from build123d import *

# Parameters (mm, degrees)
F2_R     = 9.525
F3_DEPTH = 1514.476


with BuildPart() as f1:
    # F0 (on Front) → F1 (revolve)
    with BuildSketch(Plane.XZ):
        Polygon((109.601, 15.875), (109.601, 0), (142.875, 0), (142.875, 25.4), (117.475, 25.4), (117.475, 22.225), (101.6, 22.225), (101.6, 15.875), align=None)
        Polygon((109.601, -1463.675), (109.601, 0), (109.601, 15.875), (101.6, 15.875), (101.6, -1479.55), (109.601, -1479.55), align=None)
        Polygon((144.526, -1463.675), (109.601, -1463.675), (109.601, -1479.55), (101.6, -1479.55), (101.6, -1485.9), (119.126, -1485.9), (119.126, -1489.075), (144.526, -1489.075), align=None)
    revolve(axis=Axis((0, 0, 9.743357), (0, 0, -1)))

    # F2 (on face) → F3 (cut, through all)
    with BuildSketch(Plane.XY.offset(25.4)):
        with Locations((130.175, 0)):
            Circle(F2_R)
        with Locations((112.734857, 65.0875)):
            Circle(F2_R)
        with Locations((65.0875, 112.734857)):
            Circle(F2_R)
        with Locations((0, 130.175)):
            Circle(F2_R)
        with Locations((-65.0875, 112.734857)):
            Circle(F2_R)
        with Locations((-112.734857, 65.0875)):
            Circle(F2_R)
        with Locations((-130.175, 0)):
            Circle(F2_R)
        with Locations((-112.734857, -65.0875)):
            Circle(F2_R)
        with Locations((-65.0875, -112.734857)):
            Circle(F2_R)
        with Locations((0, -130.175)):
            Circle(F2_R)
        with Locations((65.0875, -112.734857)):
            Circle(F2_R)
        with Locations((112.734857, -65.0875)):
            Circle(F2_R)
    extrude(amount=-F3_DEPTH, mode=Mode.SUBTRACT)


solid = f1.part
Can you work these out from the model? Positions are in its coordinate system, mm. A direction names the side the tool comes from. Coordinates: 2 decimals unless noted, no trailing zeros. Order: outer loops, then holes, each group sorted by start corner. A loop starts at its lowest first (then second) coordinate and runs counter-clockwise, first axis right, second up. Notation, with made-up numbers: M -11,61 L 6,61 A10 cw 6,80 Z; hole C -12,25 d8. An arc over 180 degrees is marked long. Write item = value, one per line.
(1) Suppose I cut it at B-B on x = -40.5. Please give me the cut outline in (y, z) (3 decimals).
Results are:
outline = M -138.735,-1489.075 L -112.03,-1489.075 L -112.03,-1485.9 L -93.179,-1485.9 L -93.179,22.225 L -110.273,22.225 L -110.273,25.4 L -137.015,25.4 L -137.015,0 L -101.844,0 L -101.844,-1463.675 L -138.735,-1463.675 Z; M 93.179,-1485.9 L 112.03,-1485.9 L 112.03,-1489.075 L 138.735,-1489.075 L 138.735,-1463.675 L 101.844,-1463.675 L 101.844,0 L 137.015,0 L 137.015,25.4 L 110.273,25.4 L 110.273,22.225 L 93.179,22.225 Z
(2) For faces 1 (the face through (-97, 53, -1463.675)), 2 (the face through (-93.224, 71.482, 23.79)), 3 (the face through (77.696, -121.865, -1476.197)), 4 (the face through (22, -118, -1489.075)), 5 (the face through (-88, -54, -1485.9)), which set-ups out of +Z, -Z, +X, -X, +Y, -Y let a thin tool reach every point of the face, with its end or its side?
Results are:
face_1 = none
face_2 = +Z
face_3 = +Z, -Z
face_4 = -Z, +X, -X, +Y, -Y
face_5 = -Z
(3) For pin 1 Ø4 at (x, z) = (-12.5, -1128.5) entering from -Y; pin 2 Ø3 at (x, z) = (-81.5, -291) entering from +Y; pin 3 Ø6 at (x, y) = (25, -95) entering from -Z; pin 4 Ø2 at (y, z) = (70, -969.5) entering from +X, each with a flat end and sliding along its axis, tell me the tip position at first contact or that it passes through.
Results are:
pin_1 = -109.1
pin_2 = 74.92
pin_3 = through
pin_4 = 85.16
(4) If we mould it in two halves opening along Z, with no side actions, what happens to faces 6 (the face through (-23.759, 106.995, -721.592)), 7 (the face through (113.625, -35.782, -1487.51)), 8 (the face through (-11.3, -117.1, 25.4))? For each: pulls with the +Z half, pulls with the -Z half, needs draft (parallel to the pull), parting line crosses it, or undercut.
Results are:
face_6 = undercut
face_7 = needs draft
face_8 = pulls with the +Z half
(5) Suppose I cut it at C-C on z = -1303.5. Please give me the cut outline in (x, y).
Results are:
outline = C 0,0 d219.2; hole C 0,0 d203.2
(6) I need wall thicknesses on line 1 along Y through (x, z) = (0, -1482); line 2 along Y through (x, z) = (0, 23.4) (3 decimals); line 3 along Z through (x, y) = (-100, 66) (3 decimals). Which ranges of each line are inside material? Lowest first, please. Write a range as [from, to].
Results are:
line_1 = [-144.53, -139.7], [-120.65, -101.6], [101.6, 120.65], [139.7, 144.53]
line_2 = [-142.875, -139.7], [-120.65, -117.475], [117.475, 120.65], [139.7, 142.875]
line_3 = [-1489.075, -1463.675], [0, 25.4]
(7) Suppose I cut it at A-A on y = -25.5. Please give me the cut outline in (x, z) (3 decimals).
Results are:
outline = M -142.259,-1489.075 L -116.365,-1489.075 L -116.365,-1485.9 L -98.348,-1485.9 L -98.348,22.225 L -114.674,22.225 L -114.674,25.4 L -140.581,25.4 L -140.581,0 L -106.593,0 L -106.593,-1463.675 L -142.259,-1463.675 Z; M 98.348,-1485.9 L 116.365,-1485.9 L 116.365,-1489.075 L 142.259,-1489.075 L 142.259,-1463.675 L 106.593,-1463.675 L 106.593,0 L 140.581,0 L 140.581,25.4 L 114.674,25.4 L 114.674,22.225 L 98.348,22.225 Z
